from build123d import *

# Parameters (mm, degrees)
BOX_W                  = 14
BOX_H                  = 16
BOX_DEPTH              = 10
BOX001_W               = 10
BOX001_H               = 16
BOX001_DEPTH           = 10
BOX001_PLACEMENT_ANGLE = 45


with BuildPart() as cub:
    # Box → Box (new body)
    with BuildSketch(Plane.XY):
        with Locations((7, 8)):
            Rectangle(BOX_W, BOX_H)
    extrude(amount=BOX_DEPTH)


with BuildPart() as fusion:
    # Box001 → Box001 (new body)
    with BuildSketch(Plane.XY):
        with Locations((5, 8)):
            Rectangle(BOX001_W, BOX001_H)
    extrude(amount=BOX001_DEPTH)


with BuildPart() as fusion_1:
    # Box001 placement: moved
    add(fusion.part.rotate(Axis((0, 0, 0), (0, 1, 0)), BOX001_PLACEMENT_ANGLE))

    # Fusion: union Cub
    add(cub.part)


solid = fusion_1.part
For this review, take the finished solid that the model builds, in its own axes (mm). A direction names the side the tool comes from. Give positions to 0.01 mm unless a question says otherwise; leave off trailing zeros. Loops run counter-clockwise (first coordinate to the right, second up) from the corner with the lowest first, then second, coordinate; pieces in that order, holes last. Notation, with made-up numbers: (83.25, 58) -> (103.25, 58) arc R11 ccw to (103.25, 73) -> close; hole circle Ø5 at (-32.5, 71.5). An arc over 180 degrees is marked (long way). One line per question, with ' | ' between items.
1) We need section A-A (y = 6.25). Write out the cut boundary in (x, z).
Resolved:
outline: (0, 0) -> (7.07, -7.07) -> (14.14, 0) -> (14, 0.14) -> (14, 10) -> (0, 10) -> close
2) We need section B-B (x = 3.75). Write out the cut boundary in (y, z).
Resolved:
outline: (0, -3.75) -> (16, -3.75) -> (16, 10) -> (0, 10) -> close
3) For faces 1 (the flat face through (14, 8, 5)), 2 (the flat face through (3, 8, -3)), list the 3-axis set-ups (+Z, -Z, +X, -X, +Y, -Y) from which the entire face can be reached by the end or side of a thin tool; tool diameter is ignored.
Resolved:
face 1: +Z, +X, +Y, -Y | face 2: -Z, -X, +Y, -Y
4) We need section C-C (z = -2.25). Write out the cut boundary in (x, y), plus the area to 3 significant figures.
Resolved:
outline: (2.25, 0) -> (11.89, 0) -> (11.89, 16) -> (2.25, 16) -> close | area: 154 mm2
5) Insertion check: pin 1 Ø8 at (y, z) = (5.5, 7.5) entering from +X; pin 2 Ø2 at (x, z) = (8, 3) entering from -Y; pin 3 Ø6 at (x, y) = (4.5, 3) entering from -Z. Each pin has a flat end and moves straight along its axis. Give the tip position at first contact, or say it passes through.
Resolved:
pin 1: stops at x = 14 | pin 2: stops at y = 0 | pin 3: stops at z = -7.07
6) To check wall thickness, follow probe 1 along X at (y, z) = (3, 6.25); probe 2 along Z at (x, y) = (9, 8); probe 3 along Z at (x, y) = (3.75, 15). State the ranges of each line that lie inside material, in increasing order.
Resolved:
probe 1: x = 0 to 14 | probe 2: z = -5.14 to 10 | probe 3: z = -3.75 to 10
